Geometry check sheet. Reference: the model listing, model coordinates, mm. A direction names the side the tool comes from. Round coordinates to 2 decimals unless told otherwise and drop trailing zeros. Order: outer loops, then holes, each group sorted by start corner. A loop starts at its lowest first (then second) coordinate and runs counter-clockwise, first axis right, second up. Notation, with made-up numbers: (39.25, 56.25) - (72.25, 56.25) arc R17 ccw to (72.25, 68.25) - close; hole circle Ø6 at (55, 29.25). An arc over 180 degrees is marked (long way). One line per question, with ' | ' between items. Start each with the question number.
Q1. Material ranges on line 1 along X through (y, z) = (16, -0.5); line 2 along X through (y, z) = (16, 0.5); line 3 along X through (y, z) = (8, 2.25), recorded low to high.
Q2. Mould release check, pull along Y, two halves, no side actions. Record for faces 1 (the face through (0, 2, 1)), 2 (the face through (-16.005, 13.22, -0.507)), 3 (the face through (0, 0, 0)): +Y half, -Y half, draft (parallel to the pull), parting line (faces both ways), or undercut.
Q3. Sectioned sample at B-B, the plane x = 4.5. Enter the section's corners in (y, z), then the cut area to 3 significant figures.
Q4. Gauge pin test, flat ends, axial feed: P1, Ø8, axis at x = 21, y = 11.5, coming from the -Z side; P2, Ø5, axis at x = 25, y = 20, coming from the -Z side; P3, Ø1.6, axis at y = -14, z = -2, coming from the +X side. Record the tip position at first contact, or that the pin passes through.
Q5. Tool access check on faces 4 (the face through (12.5, 13, 1)), 5 (the face through (0, -2.287, -2)), 6 (the face through (-7.423, -14, -2)), 7 (the face through (0, 0, 3)), 8 (the face through (7.001, -14, -2)). Record the directions out of +Z, -Z, +X, -X, +Y, -Y that give a thin tool (end or side, any length) a straight path to the whole face; none if there is none.
Q6. Sectioned sample at A-A, the plane y = 3.5. Enter the section's corners in (x, z), then the cut area to 3 significant figures.
Q7. Sectioned sample at D-D, the plane y = -17. Enter the section's corners in (x, z).
Q8. Sectioned sample at C-C, the plane z = 1. Give the number of separate pieces and of enclosed holes in the cut face, then the cut area to 3 significant figures.
```python
from build123d import *

# Parameters (mm, degrees)
SKETCH1_W           = 60
SKETCH1_H           = 50
BOSS_EXTRUDE1_DEPTH = 3
SKETCH2_R           = 4
CUT_EXTRUDE1_DEPTH  = 40.166312055
BOSS_EXTRUDE2_START = 1
SKETCH3_R           = 5
SKETCH3_R_2         = 4
BOSS_EXTRUDE2_DEPTH = 1
SKETCH4_W           = 25
SKETCH4_H           = 15
CUT_EXTRUDE2_DEPTH  = 40.166312055
SKETCH5_W           = 14
SKETCH5_H           = 4
CUT_EXTRUDE3_DEPTH  = 40.166312055
SKETCH6_W           = 14.423290477
SKETCH6_H           = 22.713380778
BOSS_EXTRUDE3_DEPTH = 3.3
SKETCH8_R           = 1.5
CUT_EXTRUDE4_DEPTH  = 40.190432506
SKETCH9_R           = 1.5
CUT_EXTRUDE5_DEPTH  = 10


with BuildPart() as part:
    # Sketch1 → Boss-Extrude1 (new body)
    with BuildSketch(Plane.XY):
        Rectangle(SKETCH1_W, SKETCH1_H)
    extrude(amount=BOSS_EXTRUDE1_DEPTH)

    # Sketch2 → Cut-Extrude1 (cut, through all)
    with BuildSketch(Plane(origin=(0, 0, 0), x_dir=(-1, 0, 0), z_dir=(0, 0, -1))):
        with Locations((21, 13)):
            Circle(SKETCH2_R)
        with Locations(Location((-21, 13, 0), (0, 0, 180))):
            Circle(SKETCH2_R)
    extrude(amount=-CUT_EXTRUDE1_DEPTH, mode=Mode.SUBTRACT)

    # Sketch3 → Boss-Extrude2 (add)
    # profile 1 of 2: a face of its own
    with BuildSketch(Plane(origin=(0, 0, 0), x_dir=(-1, 0, 0), z_dir=(0, 0, -1)).offset(BOSS_EXTRUDE2_START)):
        with Locations((21, 13)):
            Circle(SKETCH3_R)
        with Locations((21, 13)):
            Circle(SKETCH3_R_2, mode=Mode.SUBTRACT)
    # profile 2 of 2: a face of its own
    with BuildSketch(Plane(origin=(0, 0, 0), x_dir=(-1, 0, 0), z_dir=(0, 0, -1)).offset(BOSS_EXTRUDE2_START)):
        with Locations((-21, 13)):
            Circle(SKETCH3_R)
        with Locations((-21, 13)):
            Circle(SKETCH3_R_2, mode=Mode.SUBTRACT)
    extrude(amount=-BOSS_EXTRUDE2_DEPTH)

    # Sketch4 → Cut-Extrude2 (cut, through all)
    with BuildSketch(Plane(origin=(0, 0, 0), x_dir=(-1, 0, 0), z_dir=(0, 0, -1))):
        with Locations((0, 13.5)):
            Rectangle(SKETCH4_W, SKETCH4_H)
    extrude(amount=-CUT_EXTRUDE2_DEPTH, mode=Mode.SUBTRACT)

    # Sketch5 → Cut-Extrude3 (cut, through all)
    with BuildSketch(Plane(origin=(0, 0, 0), x_dir=(-1, 0, 0), z_dir=(0, 0, -1))):
        with Locations((0, 4)):
            Rectangle(SKETCH5_W, SKETCH5_H)
    extrude(amount=-CUT_EXTRUDE3_DEPTH, mode=Mode.SUBTRACT)

    # Sketch6 → Boss-Extrude3 (add)
    with BuildSketch(Plane(origin=(0, 0, 0), x_dir=(-1, 0, 0), z_dir=(0, 0, -1))):
        with Locations((0.211072543, -13.643309611)):
            Rectangle(SKETCH6_W, SKETCH6_H)
    extrude(amount=BOSS_EXTRUDE3_DEPTH)

    # Sketch8 → Cut-Extrude4 (cut, through all)
    with BuildSketch(Plane(origin=(0, 0, 0), x_dir=(-1, 0, 0), z_dir=(0, 0, -1))):
        with Locations((-25, 20)):
            Circle(SKETCH8_R)
        with Locations(Location((-25, -20, 0), (0, 0, 180))):
            Circle(SKETCH8_R)
        with Locations((25, -20)):
            Circle(SKETCH8_R)
        with Locations(Location((25, 20, 0), (0, 0, 180))):
            Circle(SKETCH8_R)
    extrude(amount=-CUT_EXTRUDE4_DEPTH, mode=Mode.SUBTRACT)

    # Sketch9 → Cut-Extrude5 (cut)
    with BuildSketch(Plane(origin=(0, 0, 0), x_dir=(-1, 0, 0), z_dir=(0, 0, -1))):
        with Locations((-12.000572695, -12.699531371)):
            Circle(SKETCH9_R)
        with Locations((12.000572695, -12.699531371)):
            Circle(SKETCH9_R)
    extrude(amount=-CUT_EXTRUDE5_DEPTH, mode=Mode.SUBTRACT)


solid = part.part
```
Determined:
1) line 1: x = -25 to -23.65, -18.35 to -17, 17 to 18.35, 23.65 to 25 | line 2: x = -30 to -23.65, -18.35 to -12.5, 12.5 to 18.35, 23.65 to 30 | line 3: x = -30 to -12.5, 12.5 to 30
2) face 1: undercut | face 2: parting line | face 3: draft
3) outline: (-25, -3.3) - (-2.29, -3.3) - (-2.29, 0) - (2, 0) - (2, 3) - (-25, 3) - close; (21, 0) - (25, 0) - (25, 3) - (21, 3) - close | area: 168 mm2
4) P1: stops at z = -1 | P2: stops at z = 0 | P3: stops at x = 7
5) face 4: +Z, -Z | face 5: -Z, +X, -X, +Y | face 6: -Z, -X, +Y, -Y | face 7: +Z, +X, -X, +Y, -Y | face 8: -Z, +X, +Y, -Y
6) outline: (-30, 0) - (-7, 0) - (-7, 3) - (-30, 3) - close; (7, 0) - (30, 0) - (30, 3) - (7, 3) - close | area: 138 mm2
7) outline: (-30, 0) - (-7.42, 0) - (-7.42, -3.3) - (7, -3.3) - (7, 0) - (30, 0) - (30, 3) - (-30, 3) - close
8) separate pieces: 1 | enclosed holes: 9 | area: 2,430 mm2
